Input: part model. Units: mm. Frame: model coordinates. Round coordinates to 2 decimals unless told otherwise and drop trailing zeros. Write each loop counter-clockwise with the first axis right and the second up, starting at its lowest first coordinate (ties: lowest second). Pieces come first, ordered by that corner, then holes. Notation, with made-up numbers: (23, 57.5) - (51, 57.5) arc R24 ccw to (51, 75.5) - close; hole circle Ø6 at (-34.75, -1.75). An arc over 180 degrees is marked (long way). One line per item, written item: value. Start each with the question number.
```python
from build123d import *

# Parameters (mm, degrees)
SKETCH1_W           = 100
SKETCH1_H           = 40
SKETCH1_R           = 1.5
BOSS_EXTRUDE1_DEPTH = 2


with BuildPart() as part:
    # Sketch1 → Boss-Extrude1 (new body)
    with BuildSketch(Plane.XY):
        Rectangle(SKETCH1_W, SKETCH1_H)
        with Locations((-35, -2)):
            Circle(SKETCH1_R, mode=Mode.SUBTRACT)
        with Locations(Location((35, 4, 0), (0, 0, 180))):
            Circle(SKETCH1_R, mode=Mode.SUBTRACT)
        with Locations((0, 4)):
            Circle(SKETCH1_R, mode=Mode.SUBTRACT)
        with Locations((-35, 4)):
            Circle(SKETCH1_R, mode=Mode.SUBTRACT)
        with Locations(Location((35, -2, 0), (0, 0, 180))):
            Circle(SKETCH1_R, mode=Mode.SUBTRACT)
        with Locations((0, -2)):
            Circle(SKETCH1_R, mode=Mode.SUBTRACT)
    extrude(amount=BOSS_EXTRUDE1_DEPTH)


solid = part.part
```
Q1. Cut plane B-B, the plane y = 4. Output: boundary loops of the cut face in (x, z).
Q2. Material intervals for probe 1 along Y at (x, z) = (-35, 0.7), sorted ascending. Write a range as from..to.
Q3. Contact query for a flat-ended pin moving along its axis: pin 1 Ø2.5 at (x, y) = (-35, -2) entering from -Z. Output: stop coordinate, or through.
Q4. Pull-direction query (Y, two-part tool) for faces 1 (the flat face through (-1, 0, 0)), 2 (the flat face through (-1, 20, 1)), 3 (the flat face through (-1, -20, 1)), 4 (the cylindrical face through (-36.2, -2.9, 1)); classes: pulls with the +Y half, pulls with the -Y half, needs draft (parallel to the pull), parting line crosses it, or undercut.
Q5. Cut plane A-A, the plane x = -35. Output: boundary loops of the cut face in (y, z).
A:
1. outline: (-50, 0) - (-36.5, 0) - (-36.5, 2) - (-50, 2) - close; (-33.5, 0) - (-1.5, 0) - (-1.5, 2) - (-33.5, 2) - close; (1.5, 0) - (33.5, 0) - (33.5, 2) - (1.5, 2) - close; (36.5, 0) - (50, 0) - (50, 2) - (36.5, 2) - close
2. probe 1: y = -20..-3.5, -0.5..2.5, 5.5..20
3. pin 1: passes through
4. face 1: needs draft
4. face 2: pulls with the +Y half
4. face 3: pulls with the -Y half
4. face 4: undercut
5. outline: (-20, 0) - (-3.5, 0) - (-3.5, 2) - (-20, 2) - close; (-0.5, 0) - (2.5, 0) - (2.5, 2) - (-0.5, 2) - close; (5.5, 0) - (20, 0) - (20, 2) - (5.5, 2) - close
